Check sheet for the modelled part. Datum: model origin and axes. Units: mm. Face numbers are marked on the shaded views. Round coordinates to 2 decimals unless told otherwise and drop trailing zeros. Loops run counter-clockwise (first coordinate to the right, second up) from the corner with the lowest first, then second, coordinate; pieces in that order, holes last. Notation, with made-up numbers: (10, 36.25) -> (67, 36.25) arc R7 cw to (67, 43.25) -> close; hole circle Ø9 at (10.25, 36). An arc over 180 degrees is marked (long way). One line per item, written item: value. Start each with the question number.
1. Material ranges on L1, parallel to X at y = 0, z = 45.75; L2, parallel to Y at x = 3, z = 8.5, recorded low to high.
2. Go/stop test with a flat-tipped pin: pin 1 (4 mm diameter, centred on x = 0, y = 0, fed in from +Z). Record where the tip stops, or that it passes through.
3. Release check for a two-part mould opening along X. For the marked faces 1, 2, 3 and 4 record: +X half, -X half, draft (parallel to the pull), parting line (faces both ways), or undercut.
4. Cross-section at A-A on z = 37. Record the cut outline in (x, y).
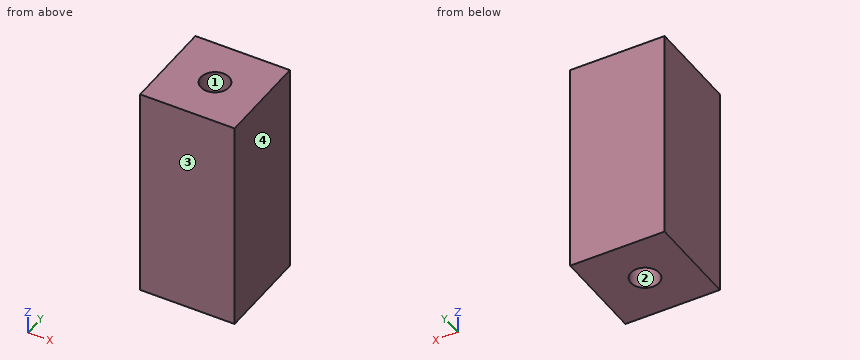
from build123d import *

# Parameters (mm, degrees)
F0_W     = 22
F0_H     = 22
F1_DEPTH = 50
F3_D     = 6.6
F3_DEPTH = 12
F3_TIP   = 1.9828400428
F5_D     = 6.6
F5_DEPTH = 12
F5_TIP   = 1.9828400428


with BuildPart() as f1:
    # F0 (on Top) → F1 (new body)
    with BuildSketch(Plane.XY):
        Rectangle(F0_W, F0_H)
    extrude(amount=F1_DEPTH)

    # F3
    with Locations(Plane.XY.offset(50)):
        with Locations((0, 0)):
            Hole(F3_D / 2, depth=F3_DEPTH)
            with Locations((0, 0, -(F3_DEPTH + F3_TIP / 2))):  # 118° drill point
                Cone(0, F3_D / 2, F3_TIP, mode=Mode.SUBTRACT)

    # F5
    with Locations(Plane(origin=(0, 0, 0), x_dir=(1, 0, 0), z_dir=(0, 0, -1))):
        with Locations((0, 0)):
            Hole(F5_D / 2, depth=F5_DEPTH)
            with Locations((0, 0, -(F5_DEPTH + F5_TIP / 2))):  # 118° drill point
                Cone(0, F5_D / 2, F5_TIP, mode=Mode.SUBTRACT)


solid = f1.part
Taken from the geometry:
1. L1: x = -11 to -3.3, 3.3 to 11
1. L2: y = -11 to -1.37, 1.37 to 11
2. pin 1: stops at z = 37.22
3. face 1: undercut
3. face 2: undercut
3. face 3: draft
3. face 4: +X half
4. outline: (-11, -11) -> (11, -11) -> (11, 11) -> (-11, 11) -> close; hole circle Ø3.27 at (0, 0)
